Source: CAD feature listing. Evaluate the final solid. Frame: model axes, mm. Face numbers are marked on the shaded views. A direction names the side the tool comes from. Round coordinates to 2 decimals unless told otherwise and drop trailing zeros. Loops run counter-clockwise (first coordinate to the right, second up) from the corner with the lowest first, then second, coordinate; pieces in that order, holes last.
(1) First-contact query: pin 1 Ø3 at (x, y) = (13, -28.5) entering from -Z; pin 2 Ø3 at (x, y) = (3.5, -6) entering from +Z. Flat tips, straight axial feed; report the tip coordinate or a pass-through.
(2) Mould query, pull axis X, two halves, no side actions, for the marked faces 4, 5 and 6. Classes: pulls with the +X half, pulls with the -X half, needs draft (parallel to the pull), parting line crosses it, or undercut.
(3) Material intervals for probe 1 along Y at (x, z) = (7.5, 1.25); probe 2 along Y at (x, z) = (4.5, 2.15); probe 3 along Y at (x, z) = (7.5, 3.8), sorted ascending.
(4) Section D-D, the plane y = -35. Return the cut outline in (x, z).
(5) Section B-B, the plane y = -21. Return the cut outline in (x, z).
(6) Section C-C, the plane x = 5.25. Return the cut outline in (y, z).
(7) Section A-A, the plane x = 7.5. Return the cut outline in (y, z), plus the area to 3 significant figures.
(8) Set-up query: the marked faces 1, 2 and 3. Return all of +Z, -Z, +X, -X, +Y, -Y with unobstructed straight access to the full face (end or side cutting, diameter ignored); none if empty.
```python
from build123d import *

# Parameters (mm, degrees)
SKETCH1_W                 = 15
SKETCH1_H                 = 40
BOSS_EXTRUDE1_DEPTH       = 5
CUT_EXTRUDE1_DEPTH        = 3
CUT_EXTRUDE2_DEPTH        = 3
CUT_EXTRUDE3_DEPTH        = 3
CUT_EXTRUDE4_DEPTH        = 6
F_4_CLEARANCE_HOLE1_D     = 3.3
F_4_CLEARANCE_HOLE1_DEPTH = 5
FILLET1_R                 = 3


with BuildPart() as part:
    # Sketch1 → Boss-Extrude1 (new body)
    with BuildSketch(Plane.XY.offset(5)):
        with Locations((7.5, -20)):
            Rectangle(SKETCH1_W, SKETCH1_H)
    extrude(amount=-BOSS_EXTRUDE1_DEPTH)

    # Sketch2 → Cut-Extrude1 (cut)
    with BuildSketch(Plane.XY.offset(5)):
        with BuildLine():
            Line((0, -8.25), (10.5, -8.25))
            ThreePointArc((10.5, -8.25), (13.75, -5), (10.5, -1.75))
            Line((10.5, -1.75), (0, -1.75))
            Line((0, -1.75), (0, -8.25))
        make_face()
    extrude(amount=-CUT_EXTRUDE1_DEPTH, mode=Mode.SUBTRACT)

    # Sketch3 → Cut-Extrude2 (cut, through all)
    with BuildSketch(Plane.XY.offset(2)):
        with BuildLine():
            Line((0, -3.3), (0, -6.7))
            Line((0, -6.7), (10.5, -6.7))
            ThreePointArc((10.5, -6.7), (12.2, -5), (10.5, -3.3))
            Line((10.5, -3.3), (0, -3.3))
        make_face()
    extrude(amount=-CUT_EXTRUDE2_DEPTH, mode=Mode.SUBTRACT)

    # Sketch4 → Cut-Extrude3 (cut)
    with BuildSketch(Plane.XY.offset(5)):
        with BuildLine():
            Line((0, -38.25), (10.5, -38.25))
            ThreePointArc((10.5, -38.25), (13.75, -35), (10.5, -31.75))
            Line((10.5, -31.75), (0, -31.75))
            Line((0, -31.75), (0, -38.25))
        make_face()
    extrude(amount=-CUT_EXTRUDE3_DEPTH, mode=Mode.SUBTRACT)

    # Sketch5 → Cut-Extrude4 (cut, through all)
    with BuildSketch(Plane(origin=(0, 0, 0), x_dir=(-1, 0, 0), z_dir=(0, 0, -1))):
        with BuildLine():
            Line((0, -36.75), (0, -33.25))
            Line((0, -33.25), (-10.5, -33.25))
            ThreePointArc((-10.5, -33.25), (-12.25, -35), (-10.5, -36.75))
            Line((-10.5, -36.75), (0, -36.75))
        make_face()
    extrude(amount=-CUT_EXTRUDE4_DEPTH, mode=Mode.SUBTRACT)

    # #4 Clearance Hole1
    with Locations(Plane.XY.offset(5)):
        with Locations((7.5, -20)):
            Hole(F_4_CLEARANCE_HOLE1_D / 2, depth=F_4_CLEARANCE_HOLE1_DEPTH)

    # Fillet1
    fillet1_edges = [part.edges().sort_by_distance(p)[0] for p in [
        (15, -40, 2.5),
        (15, 0, 2.5),
    ]]
    fillet(fillet1_edges, radius=FILLET1_R)


solid = part.part
```
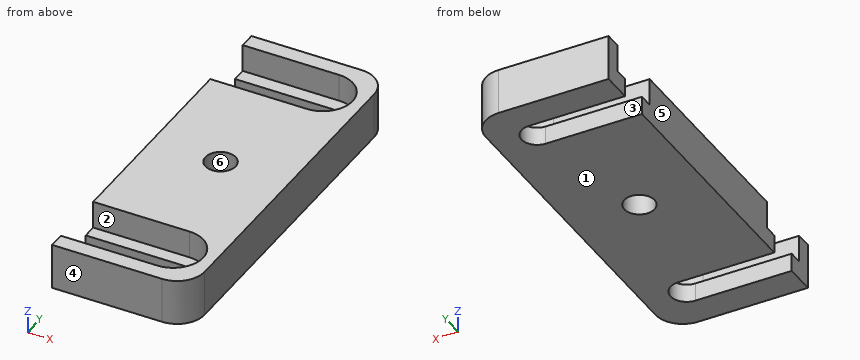
Output values:
1. pin 1: stops at z = 0
1. pin 2: stops at z = 2
2. face 4: needs draft
2. face 5: pulls with the -X half
2. face 6: undercut
3. probe 1: y = -40 to -36.75, -33.25 to -21.65, -18.35 to -6.7, -3.3 to 0
3. probe 2: y = -40 to -38.25, -31.75 to -8.25, -1.75 to 0
3. probe 3: y = -40 to -38.25, -31.75 to -21.65, -18.35 to -8.25, -1.75 to 0
4. outline: (12.25, 0) - (15, 0) - (15, 5) - (13.75, 5) - (13.75, 2) - (12.25, 2) - close
5. outline: (0, 0) - (6.19, 0) - (6.19, 5) - (0, 5) - close; (8.81, 0) - (15, 0) - (15, 5) - (8.81, 5) - close
6. outline: (-40, 0) - (-36.75, 0) - (-36.75, 2) - (-38.25, 2) - (-38.25, 5) - (-40, 5) - close; (-33.25, 0) - (-6.7, 0) - (-6.7, 2) - (-8.25, 2) - (-8.25, 5) - (-31.75, 5) - (-31.75, 2) - (-33.25, 2) - close; (-3.3, 0) - (0, 0) - (0, 5) - (-1.75, 5) - (-1.75, 2) - (-3.3, 2) - close
7. outline: (-40, 0) - (-36.75, 0) - (-36.75, 2) - (-38.25, 2) - (-38.25, 5) - (-40, 5) - close; (-33.25, 0) - (-21.65, 0) - (-21.65, 5) - (-31.75, 5) - (-31.75, 2) - (-33.25, 2) - close; (-18.35, 0) - (-6.7, 0) - (-6.7, 2) - (-8.25, 2) - (-8.25, 5) - (-18.35, 5) - close; (-3.3, 0) - (0, 0) - (0, 5) - (-1.75, 5) - (-1.75, 2) - (-3.3, 2) - close
7. area: 131 mm2
8. face 1: -Z, +X, -X, +Y, -Y
8. face 2: +Z, -X
8. face 3: +Z, -Z, -X
